from build123d import *

# Parameters (mm, degrees)
F0_W      = 127
F0_H      = 76
F1_DEPTH  = 200
F3_DEPTH  = 76.001
F4_W      = 26
F4_H      = 26
F6_W      = 76
F6_H      = 26
F7_DEPTH  = 76
F8_R      = 37.99999
F9_W      = 76
F9_H      = 26
F10_DEPTH = 76
F11_R     = 37.99999
F12_R     = 19
F13_DEPTH = 26.001
F12_R_2   = 28.5
F14_DEPTH = 1
F15_R     = 6
F16_R     = 28.5
F16_R_2   = 19
F17_DEPTH = 1
F18_DEPTH = 26


# Not quite as in the source:
# - a fillet or chamfer is up to 0.001 mm smaller than in the source, because OpenCascade refuses the exact size
# - a feature names something its author has since deleted; it is built from what else it names


with BuildPart() as f1:
    # F0 (on Top) → F1 (new body)
    with BuildSketch(Plane.XY):
        with Locations((63.5, 38)):
            Rectangle(F0_W, F0_H)
    extrude(amount=F1_DEPTH)

    # F2 (on face) → F3 (cut, through all)
    with BuildSketch(Plane.XZ):
        Polygon((38, 139), (127, 50), (127, 200), (0, 200), (0, 177), align=None)
        Polygon((0, 139), (38, 139), (0, 177), align=None)
    extrude(amount=-F3_DEPTH, mode=Mode.SUBTRACT)

    # F5: sweep along a path in F2
    with BuildLine(Plane.XZ) as f5_path:
        Line((0, 177), (191.2105315588, -14.2105315588))
    # F4 (on face) → F5 (sweep, cut)
    with BuildSketch(Plane.XY.offset(139)):
        with Locations((25, 39)):
            Rectangle(F4_W, F4_H)
    sweep(path=f5_path.line, mode=Mode.SUBTRACT)

    # F6 (on face) → F7 (join)
    with BuildSketch(Plane.XZ):
        with Locations((38, 13)):
            Rectangle(F6_W, F6_H)
    extrude(amount=F7_DEPTH)

    # F8 (radius 38 in the source; OpenCascade refuses exactly that, so slightly less here)
    f8_edges = [f1.edges().sort_by_distance(p)[0] for p in [
        (76, -76, 13),
        (0, -76, 13),
    ]]
    fillet(f8_edges, radius=F8_R)

    # F9 (on face) → F10 (join)
    with BuildSketch(Plane(origin=(0, 76, 0), x_dir=(-1, 0, 0), z_dir=(0, 1, 0))):
        with Locations((-38, 13)):
            Rectangle(F9_W, F9_H)
    extrude(amount=F10_DEPTH)

    # F11 (radius 38 in the source; OpenCascade refuses exactly that, so slightly less here)
    f11_edges = [f1.edges().sort_by_distance(p)[0] for p in [
        (0, 152, 13),
        (76, 152, 13),
    ]]
    fillet(f11_edges, radius=F11_R)

    # F12 (on face) → F13 (cut, through all)
    with BuildSketch(Plane.XY.offset(26)):
        with Locations((38, 114)):
            Circle(F12_R)
    extrude(amount=-F13_DEPTH, mode=Mode.SUBTRACT)

    # F12 (on face) → F14 (cut)
    with BuildSketch(Plane.XY.offset(26)):
        with Locations((38, 114)):
            Circle(F12_R_2)
        with Locations((38, 114)):
            Circle(F12_R, mode=Mode.SUBTRACT)
    extrude(amount=-F14_DEPTH, mode=Mode.SUBTRACT)

    # F15
    f15_edges = [f1.edges().sort_by_distance(p)[0] for p in [
        (64.870061, 140.870061, 26),
        (11.129939, -64.870061, 26),
    ]]
    fillet(f15_edges, radius=F15_R)

    # F16 (on face) → F17 (cut)
    with BuildSketch(Plane.XY.offset(26)):
        with Locations((38, -38)):
            Circle(F16_R)
        with Locations((38, -38)):
            Circle(F16_R_2, mode=Mode.SUBTRACT)
    extrude(amount=-F17_DEPTH, mode=Mode.SUBTRACT)

    # F18 (cut, through all): a face of the model
    f18_faces = [f1.faces().sort_by_distance(p)[0] for p in [
        (38, -38, 26),
    ]]
    extrude(f18_faces, amount=-F18_DEPTH, mode=Mode.SUBTRACT)


solid = f1.part
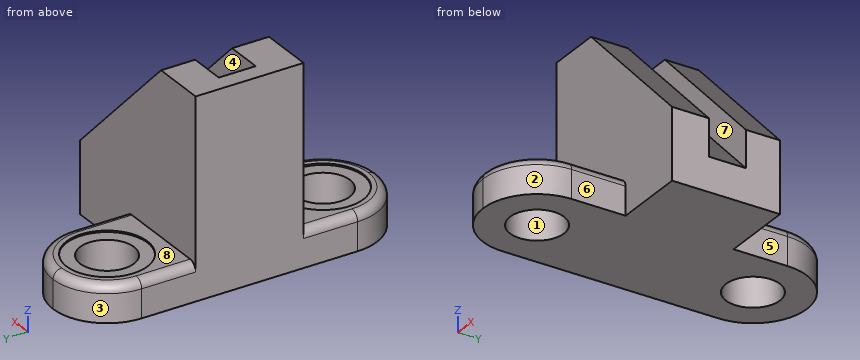
Geometry check sheet. Reference: the model listing, model coordinates, mm. Face numbers are marked on the shaded views. A direction names the side the tool comes from. Round coordinates to 2 decimals unless told otherwise and drop trailing zeros. Loops run counter-clockwise (first coordinate to the right, second up) from the corner with the lowest first, then second, coordinate; pieces in that order, holes last. Notation, with made-up numbers: (-14.75, 25) - (7.25, 25) arc R6 cw to (7.25, 32) - close; hole circle Ø4 at (46.25, 13). An arc over 180 degrees is marked (long way). One line per question, with ' | ' between items. Start each with the question number.
1. Draft check along X on the marked faces 1, 2, 3 and 4. Enter one of: released by +X, released by -X, zero draft, split by the parting line, or undercut.
2. Cross-section at C-C on x = 115. Record the cut outline in (y, z).
3. Cross-section at B-B on z = 61.5. Record the cut outline in (x, y), then the cut area to 3 significant figures.
4. Depth check by flat-ended pin: pin 1 (1.5 mm diameter, centred on x = 113, y = 70, fed in from +Z); pin 2 (10 mm diameter, centred on x = 26, z = 117.5, fed in from -Y); pin 3 (6 mm diameter, centred on y = -27, z = 5.5, fed in from +X); pin 4 (23 mm diameter, centred on x = 38, y = 114, fed in from +Z). Enter the tip coordinate at first touch or a pass-through.
5. Tool access check on the marked faces 5, 6, 7 and 8. Record the directions out of +Z, -Z, +X, -X, +Y, -Y that give a thin tool (end or side, any length) a straight path to the whole face; none if there is none.
6. Cross-section at A-A on y = 111.5. Record the cut outline in (x, z).
7. Scan lines: line 1 (Y direction, x = 70, z = 97); line 2 (Y direction, x = 92, z = 10.5); line 3 (Z direction, x = 40, y = 87). Record each from-to range of solid material in increasing order. Write a range as [from, to].
8. Cross-section at D-D on y = 58. Record the cut outline in (x, z), then the cut area to 3 significant figures.
Taken from the geometry:
1) face 1: undercut | face 2: released by +X | face 3: released by -X | face 4: zero draft
2) outline: (0, 0) - (76, 0) - (76, 62) - (52, 62) - (52, 36) - (26, 36) - (26, 62) - (0, 62) - close
3) outline: (0, 0) - (115.5, 0) - (115.5, 26) - (89.5, 26) - (89.5, 52) - (115.5, 52) - (115.5, 76) - (0, 76) - close | area: 8,100 mm²
4) pin 1: z = 64.75 | pin 2: y = 0 | pin 3: x = 76 | pin 4: through
5) face 5: +Z, -Z, +X, +Y | face 6: +Z, -Z, +X, -Y | face 7: +Z, +X | face 8: +Z, +X, -X, +Y
6) outline: (0, 0) - (19.17, 0) - (19.17, 25) - (9.61, 25) - (9.61, 26) - (6, 26) arc R6 ccw to (0, 20) - close; (56.83, 0) - (76, 0) - (76, 20) arc R6 ccw to (70, 26) - (66.39, 26) - (66.39, 25) - (56.83, 25) - close
7) line 1: [0, 26], [52, 76] | line 2: [0, 76] | line 3: [0, 25]
8) outline: (0, 0) - (127, 0) - (127, 50) - (38, 139) - (0, 139) - close | area: 13,700 mm²
